```python
from build123d import *

# Parameters (mm, degrees)
SKETCH_2_R           = 32.5
EXTRUDE_1_DEPTH      = 3
EXTRUDE_START        = 43.5
SKETCH_3_R           = 32.5
SKETCH_3_R_2         = 30.5
EXTRUDE_2_DEPTH      = 43.5
SKETCH_4_W           = 35
SKETCH_4_H           = 18.5
CUT_EXTRUDE_1_DEPTH  = 52
EXTRUDE_3_REACH      = 93.83
EXTRUDE_3_END_RADIUS = 30.5
SKETCH_5_W           = 41
SKETCH_5_H           = 22.5
SKETCH_5_W_2         = 35
SKETCH_5_H_2         = 18.5
SKETCH_9_W           = 43.61428081
SKETCH_9_H           = 23.224697296
CUT_EXTRUDE_2_DEPTH  = 2
EXTRUDE_4_DEPTH      = 22.5
SKETCH_11_W          = 18.5
SKETCH_11_H          = 36.291622976
CUT_REVOLVE_1_ANGLE  = 15
SKETCH_12_W          = 18.5
SKETCH_12_H          = 37.014975327
CUT_REVOLVE_2_ANGLE  = 15
CUT_REVOLVE_3_ANGLE  = 5
CUT_REVOLVE_4_ANGLE  = 5
EXTRUDE_START_2      = 3
EXTRUDE_5_DEPTH      = 3
SKETCH_17_W          = 36.670628391
SKETCH_17_H          = 24.683517756
CUT_EXTRUDE_3_DEPTH  = 3
CHAMFER_1_SIZE       = 4
FILLET_1_R           = 1
EXTRUDE_6_REACH      = 67.382
SKETCH_18_R          = 3
SKETCH_19_R          = 3
EXTRUDE_7_DEPTH      = 18
SKETCH_20_R          = 0.95
CUT_EXTRUDE_4_DEPTH  = 10
SKETCH_21_R          = 44.197984087
CUT_EXTRUDE_5_DEPTH  = 2


with BuildPart() as part:
    # 草图2 → 凸台-拉伸1 (new body)
    with BuildSketch(Plane.XY.offset(76.5)):
        Circle(SKETCH_2_R)
    extrude(amount=EXTRUDE_1_DEPTH)

    # 草图3 → 凸台-拉伸2 (add)
    with BuildSketch(Plane(origin=(0, 0, 76.5), x_dir=(-1, 0, 0), z_dir=(0, 0, -1)).offset(EXTRUDE_START)):
        Circle(SKETCH_3_R)
        Circle(SKETCH_3_R_2, mode=Mode.SUBTRACT)
    extrude(amount=-EXTRUDE_2_DEPTH)

    # 草图4 → 切除-拉伸1 (cut)
    with BuildSketch(Plane(origin=(0, 0, 0), x_dir=(1, 0, 0), z_dir=(0, 1, 0))):
        with Locations((0, -65.25)):
            Rectangle(SKETCH_4_W, SKETCH_4_H)
    extrude(amount=CUT_EXTRUDE_1_DEPTH, mode=Mode.SUBTRACT)

    # 凸台-拉伸3: up to this cylinder (the profile starts inside it)
    extrude_3_end = Plane(origin=(0, 0, 54.46768), z_dir=(0, 0, 1)) * Cylinder(EXTRUDE_3_END_RADIUS, 249.66, mode=Mode.PRIVATE)
    # 草图5 → 凸台-拉伸3 (add, up to the surface)
    with BuildSketch(Plane(origin=(0, 0, 0), x_dir=(1, 0, 0), z_dir=(0, 1, 0)), mode=Mode.PRIVATE) as extrude_3_sk1:
        with Locations((0, -65.25)):
            Rectangle(SKETCH_5_W, SKETCH_5_H)
        with Locations((0, -65.25)):
            Rectangle(SKETCH_5_W_2, SKETCH_5_H_2, mode=Mode.SUBTRACT)
    extrude_3_tool1 = extrude(extrude_3_sk1.sketch, amount=EXTRUDE_3_REACH, mode=Mode.PRIVATE) & extrude_3_end
    add(extrude_3_tool1.solids().sort_by_distance((0, 0, 54.46768))[0])

    # 草图9 → 切除-拉伸2 (cut)
    with BuildSketch(Plane.XZ):
        with Locations((0, 64.887651352)):
            Rectangle(SKETCH_9_W, SKETCH_9_H)
    extrude(amount=-CUT_EXTRUDE_2_DEPTH, mode=Mode.SUBTRACT)

    # 草图10 → 凸台-拉伸4 (add)
    with BuildSketch(Plane(origin=(0, 0, 54), x_dir=(-1, 0, 0), z_dir=(0, 0, -1))):
        with BuildLine():
            Line((20.5, 2), (30.434355587, 2))
            ThreePointArc((30.434355587, 2), (27.468053538, 13.257301189), (20.5, 22.583179581))
            Line((20.5, 22.583179581), (20.5, 2))
        make_face()
        with BuildLine():
            Line((-20.5, 2), (-30.434355587, 2))
            ThreePointArc((-30.434355587, 2), (-27.468053538, 13.257301189), (-20.5, 22.583179581))
            Line((-20.5, 22.583179581), (-20.5, 2))
        make_face()
    extrude(amount=-EXTRUDE_4_DEPTH)

    # 草图11 → 切除-旋转1 (revolve, cut)
    with BuildSketch(Plane.ZY.offset(-17.5)):
        with Locations((65.25, 20.145811488)):
            Rectangle(SKETCH_11_W, SKETCH_11_H)
    revolve(axis=Axis((17.5, 2, 81.98075626), (0, 0, -1)), revolution_arc=CUT_REVOLVE_1_ANGLE, mode=Mode.SUBTRACT)

    # 草图12 → 切除-旋转2 (revolve, cut)
    with BuildSketch(Plane(origin=(-17.5, 0, 0), x_dir=(0, 0, -1), z_dir=(1, 0, 0))):
        with Locations((-65.25, 20.507487664)):
            Rectangle(SKETCH_12_W, SKETCH_12_H)
    revolve(axis=Axis((-17.5, 2, 82.239096386), (0, 0, 1)), revolution_arc=CUT_REVOLVE_2_ANGLE, mode=Mode.SUBTRACT)

    # 草图13 → 切除-旋转3 (revolve, cut)
    with BuildSketch(Plane.XY.offset(56)):
        Polygon((-17.5, 2), (17.5, 2), (26.341893189, 34.998394615), (-26.341893189, 34.998394615), align=None)
    revolve(axis=Axis((-38.580818274, 2, 56), (-1, 0, 0)), revolution_arc=CUT_REVOLVE_3_ANGLE, mode=Mode.SUBTRACT)

    # 草图14 → 切除-旋转4 (revolve, cut)
    with BuildSketch(Plane(origin=(0, 0, 74.5), x_dir=(-1, 0, 0), z_dir=(0, 0, -1))):
        Polygon((17.5, 2), (-17.5, 2), (-26.592656258, 35.805125046), (26.592656258, 35.805125046), align=None)
    revolve(axis=Axis((-42.793281967, 2, 74.5), (1, 0, 0)), revolution_arc=CUT_REVOLVE_4_ANGLE, mode=Mode.SUBTRACT)

    # 草图15 → 凸台-拉伸5 (add)
    with BuildSketch(Plane(origin=(0, 0, 54), x_dir=(-1, 0, 0), z_dir=(0, 0, -1)).offset(EXTRUDE_START_2)):
        with BuildLine():
            Line((30.434355587, 2), (-30.434355587, 2))
            ThreePointArc((-30.434355587, 2), (0, 30.5), (30.434355587, 2))
        make_face()
    extrude(amount=-EXTRUDE_5_DEPTH)

    # 草图17 → 切除-拉伸3 (cut)
    with BuildSketch(Plane(origin=(0, 4.877341222, 55.748265262), x_dir=(1, 0, 0), z_dir=(0, 0.08715574274765839, 0.9961946980917457))):
        with Locations((0.24825377, 21.222934692)):
            Rectangle(SKETCH_17_W, SKETCH_17_H)
    extrude(amount=CUT_EXTRUDE_3_DEPTH, mode=Mode.SUBTRACT)

    # 倒角1
    chamfer_1_edges = [part.edges().sort_by_distance(p)[0] for p in [
        (0, 2, 51),
    ]]
    chamfer(chamfer_1_edges, length=CHAMFER_1_SIZE)

    # 圆角1
    fillet_1_edges = [part.edges().sort_by_distance(p)[0] for p in [
        (-32.5, 0, 79.5),
    ]]
    fillet(fillet_1_edges, radius=FILLET_1_R)

    # 凸台-拉伸6: up to this face of the body (flat: up to its plane)
    extrude_6_end = Plane(part.part.faces().sort_by_distance((0, -11.870804721, 76.5))[0])
    # 草图18 → 凸台-拉伸6 (add, up to the picked face)
    with BuildSketch(Plane(origin=(0, 0, 33), x_dir=(-1, 0, 0), z_dir=(0, 0, -1)), mode=Mode.PRIVATE) as extrude_6_sk1:
        with Locations((-29.5, 0)):
            Circle(SKETCH_18_R)
    extrude_6_tool1 = split(extrude(extrude_6_sk1.sketch, amount=-EXTRUDE_6_REACH, mode=Mode.PRIVATE), bisect_by=extrude_6_end, keep=Keep.BOTH, mode=Mode.PRIVATE)
    # 草图18 → 凸台-拉伸6 (add, up to the picked face)
    with BuildSketch(Plane(origin=(0, 0, 33), x_dir=(-1, 0, 0), z_dir=(0, 0, -1)), mode=Mode.PRIVATE) as extrude_6_sk2:
        with Locations((0, -29.5)):
            Circle(SKETCH_18_R)
    extrude_6_tool2 = split(extrude(extrude_6_sk2.sketch, amount=-EXTRUDE_6_REACH, mode=Mode.PRIVATE), bisect_by=extrude_6_end, keep=Keep.BOTH, mode=Mode.PRIVATE)
    # 草图18 → 凸台-拉伸6 (add, up to the picked face)
    with BuildSketch(Plane(origin=(0, 0, 33), x_dir=(-1, 0, 0), z_dir=(0, 0, -1)), mode=Mode.PRIVATE) as extrude_6_sk3:
        with Locations((29.5, 0)):
            Circle(SKETCH_18_R)
    extrude_6_tool3 = split(extrude(extrude_6_sk3.sketch, amount=-EXTRUDE_6_REACH, mode=Mode.PRIVATE), bisect_by=extrude_6_end, keep=Keep.BOTH, mode=Mode.PRIVATE)
    add(extrude_6_tool1.solids().sort_by(Axis((29.5, 0, 33), (0, 0, 1)))[0])
    add(extrude_6_tool2.solids().sort_by(Axis((0, -29.5, 33), (0, 0, 1)))[0])
    add(extrude_6_tool3.solids().sort_by(Axis((-29.5, 0, 33), (0, 0, 1)))[0])

    # 草图19 → 凸台-拉伸7 (add)
    with BuildSketch(Plane(origin=(0, 0, 33), x_dir=(-1, 0, 0), z_dir=(0, 0, -1))):
        with Locations((0, 29.5)):
            Circle(SKETCH_19_R)
    extrude(amount=-EXTRUDE_7_DEPTH)

    # 草图20 → 切除-拉伸4 (cut)
    with BuildSketch(Plane(origin=(0, 0, 33), x_dir=(-1, 0, 0), z_dir=(0, 0, -1))):
        with Locations((0, -29.5)):
            Circle(SKETCH_20_R)
        with Locations((29.5, 0)):
            Circle(SKETCH_20_R)
        with Locations((0, 29.5)):
            Circle(SKETCH_20_R)
        with Locations((-29.5, 0)):
            Circle(SKETCH_20_R)
    extrude(amount=-CUT_EXTRUDE_4_DEPTH, mode=Mode.SUBTRACT)

    # 草图21 → 切除-拉伸5 (cut)
    with BuildSketch(Plane(origin=(0, 0, 33), x_dir=(-1, 0, 0), z_dir=(0, 0, -1))):
        Circle(SKETCH_21_R)
    extrude(amount=-CUT_EXTRUDE_5_DEPTH, mode=Mode.SUBTRACT)


solid = part.part
```
CAD build for the part. Positions are in the model's coordinates, mm. A direction names the side the tool comes from. Round coordinates to 2 decimals unless told otherwise and drop trailing zeros. Write each loop counter-clockwise with the first axis right and the second up, starting at its lowest first coordinate (ties: lowest second). Pieces come first, ordered by that corner, then holes. Notation, with made-up numbers: (-32.75, 33) -> (19.25, 33) arc R18 ccw to (19.25, 40) -> close; hole circle Ø11 at (23, 70). An arc over 180 degrees is marked (long way). Answer in a Markdown table with one row per item. Add a question column.
Item 1: Drill centre lines: line 1 (Y direction, x = 0, z = 40); line 2 (Z direction, x = -19.5, y = 23); line 3 (Z direction, x = 17.5, y = -7.5). Where is each one in solid material? Low to high. Write a range as from..to.
Item 2: Drop flat-ended pins along their axis: pin 1 Ø1.5 at (x, z) = (-14, 58.5) entering from -Y; pin 2 Ø3 at (y, z) = (19.5, 47) entering from +X; pin 3 Ø3 at (x, z) = (-17, 59) entering from -Y. Give the stop position or say it passes through.
Item 3: Saw through at D-D, the plane z = 73. Write the cut outline in (x, y), then the cut area to 3 significant figures.
Item 4: Saw through at B-B, the plane z = 48. Write the cut outline in (x, y).
Item 5: Which spindle directions (+Z, -Z, +X, -X, +Y, -Y) get a long thin tool onto all of the face, cutting with end or side? Do faces 4 (the face through (-0.324, 17.464, 54.647)), 5 (the face through (0.206, 28.573, 38.944)). Say none if no direction does.
Item 6: Mould opens along X. For faces 1 (the face through (30.45, 0.04, 38.94)), 2 (the face through (0, 27, 35)), 3 (the face through (-2.14, 32.43, 51.61)) say: pulls with the +X half, pulls with the -X half, needs draft (parallel to the pull), parting line crosses it, or undercut.
Item 7: Saw through at A-A, the plane x = 0. Write the cut outline in (y, z), then the cut area to 3 significant figures.
Item 8: Saw through at C-C, the plane y = 0. Write the cut outline in (x, z), then the cut area to 3 significant figures.
Findings below:
| question | item | result |
|---|---|---|
| 1 | line 1 | y = -32.5..-30.45, -28.55..-26.5, 26.5..28.55, 30.45..32.5 |
| 1 | line 2 | z = 51..54.16, 76.34..79.5 |
| 1 | line 3 | z = 76.5..79.5 |
| 2 | pin 1 | stops at y = -29.68 |
| 2 | pin 2 | stops at x = 27.06 |
| 2 | pin 3 | stops at y = -28.57 |
| 3 | outline | (-30.36, -2.87) arc R3 ccw to (-27.26, 2) -> (-17.5, 2) -> (-23.09, 22.87) arc R32.5 ccw (long way) to (23.09, 22.87) -> (17.5, 2) -> (27.26, 2) arc R3 ccw to (30.36, -2.87) arc R30.5 cw to (2.87, -30.36) arc R3 ccw (long way) to (-2.87, -30.36) arc R30.5 cw to start |
| 3 | area | 636 mm^2 |
| 4 | outline | circle Ø65 at (0, 0); hole (-30.36, -2.87) arc R30.5 ccw to (-2.87, -30.36) arc R3 cw (long way) to (2.87, -30.36) arc R30.5 ccw to (30.36, -2.87) arc R3 cw (long way) to (30.36, 2.87) arc R30.5 ccw to (2.87, 30.36) arc R3 cw (long way) to (-2.87, 30.36) arc R30.5 ccw to (-30.36, 2.87) arc R3 cw (long way) to start |
| 5 | face 4 | +Y |
| 5 | face 5 | -Z |
| 6 | face 1 | undercut |
| 6 | face 2 | needs draft |
| 6 | face 3 | parting line crosses it |
| 7 | outline | (-32.5, 35) -> (-30.45, 35) -> (-30.45, 43) -> (-28.55, 43) -> (-28.55, 35) -> (-26.5, 35) -> (-26.5, 76.5) -> (2, 76.5) -> (2, 74.5) -> (32.5, 77.17) -> (32.5, 78.5) arc R1 ccw to (31.5, 79.5) -> (-31.5, 79.5) arc R1 ccw to (-32.5, 78.5) -> close; (2, 55) -> (6, 51) -> (26.5, 51) -> (26.5, 35) -> (28.55, 35) -> (28.55, 43) -> (30.45, 43) -> (30.45, 35) -> (32.5, 35) -> (32.5, 53.33) -> (2, 56) -> close |
| 7 | area | 633 mm^2 |
| 8 | outline | (-32.5, 35) -> (-30.45, 35) -> (-30.45, 43) -> (-28.55, 43) -> (-28.55, 35) -> (-26.5, 35) -> (-26.5, 76.5) -> (26.5, 76.5) -> (26.5, 35) -> (28.55, 35) -> (28.55, 43) -> (30.45, 43) -> (30.45, 35) -> (32.5, 35) -> (32.5, 78.5) arc R1 ccw to (31.5, 79.5) -> (-31.5, 79.5) arc R1 ccw to (-32.5, 78.5) -> close |
| 8 | area | 662 mm^2 |
